Check sheet for the drawn part. Datum: minimum x, y, z corner. Units: mm. Give positions to 0.01 mm unless a question says otherwise; leave off trailing zeros. Order: outer loops, then holes, each group sorted by start corner. A loop starts at its lowest first (then second) coordinate and runs counter-clockwise, first axis right, second up. Notation, with made-up numbers: (69.25, 57.5) - (104.25, 57.5) arc R36 ccw to (104.25, 91.5) - close; hole circle Ø6 at (28, -16.75). An arc over 180 degrees is marked (long way). Answer as a JSON object with one key per item and string values. Group by question number.
(1) Thickness scan on line 1 (Y direction, x = 54.26, z = 2.4); line 2 (X direction, y = 12.5, z = 3.1); line 3 (Y direction, x = 111.78, z = 2.1). Record the ranges inside material, lowest first.
(2) Section check D-D (y = 13.93). Record the boundary of the cut face in (x, z).
(3) Section check A-A (z = 1.6). Count the separate pieces of the cut face and the enclosed holes in it, then the cut area to 3 significant figures.
(4) Depth check by flat-ended pin: pin 1 Ø3 at (x, z) = (33, 2.5) entering from +Y; pin 2 Ø3 at (x, z) = (124, 4.5) entering from -Y. Enter the tip coordinate at first touch or a pass-through.
(5) Section check C-C (y = 128.81). Record the boundary of the cut face in (x, z), then the cut area to 3 significant figures.
(6) Section check B-B (x = 54.26). Record the boundary of the cut face in (y, z), then the cut area to 3 significant figures.
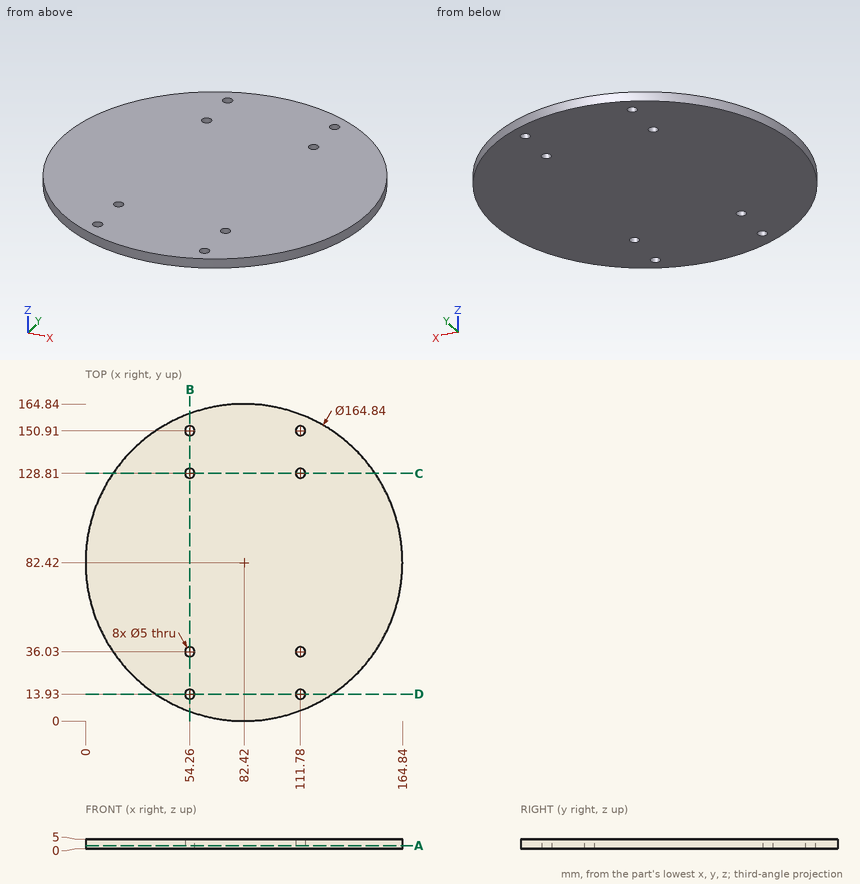
Solutions:
{
 "1": {"line 1": "y = 4.96 to 11.43, 16.43 to 33.53, 38.53 to 126.31, 131.31 to 148.41, 153.41 to 159.88", "line 2": "x = 38.78 to 52.21, 56.31 to 109.73, 113.83 to 126.06", "line 3": "y = 5.41 to 11.43, 16.43 to 33.53, 38.53 to 126.31, 131.31 to 148.41, 153.41 to 159.43"},
 "2": {"outline": "(36.57, 0) - (51.76, 0) - (51.76, 5) - (36.57, 5) - close; (56.76, 0) - (109.28, 0) - (109.28, 5) - (56.76, 5) - close; (114.28, 0) - (128.27, 0) - (128.27, 5) - (114.28, 5) - close"},
 "3": {"separate pieces": "1", "enclosed holes": "8", "area": "21,200 mm2"},
 "4": {"pin 1": "stops at y = 149.48", "pin 2": "stops at y = 10.4"},
 "5": {"outline": "(14.29, 0) - (51.76, 0) - (51.76, 5) - (14.29, 5) - close; (56.76, 0) - (109.28, 0) - (109.28, 5) - (56.76, 5) - close; (114.28, 0) - (150.55, 0) - (150.55, 5) - (114.28, 5) - close", "area": "631 mm2"},
 "6": {"outline": "(4.96, 0) - (11.43, 0) - (11.43, 5) - (4.96, 5) - close; (16.43, 0) - (33.53, 0) - (33.53, 5) - (16.43, 5) - close; (38.53, 0) - (126.31, 0) - (126.31, 5) - (38.53, 5) - close; (131.31, 0) - (148.41, 0) - (148.41, 5) - (131.31, 5) - close; (153.41, 0) - (159.88, 0) - (159.88, 5) - (153.41, 5) - close", "area": "675 mm2"}
}
